Input: dimensioned drawing with shaded views. Units: mm. Origin: part minimum x, y, z. A direction names the side the tool comes from. Round coordinates to 2 decimals unless told otherwise and drop trailing zeros. Order: outer loops, then holes, each group sorted by start corner. A loop starts at its lowest first (then second) coordinate and runs counter-clockwise, first axis right, second up.
Item 1: First-contact query: pin 1 (6 mm diameter, centred on y = 36, z = 19.5, fed in from -X); pin 2 (1.5 mm diameter, centred on x = 41, z = 11.5, fed in from +Y); pin 3 (10 mm diameter, centred on y = 36.5, z = 24.5, fed in from +X); pin 4 (10.5 mm diameter, centred on x = 21.5, z = 13, fed in from +Y). Flat tips, straight axial feed; report the tip coordinate or a pass-through.
Item 2: Cut plane B-B on x = 50. Output: boundary loops of the cut face in (y, z).
Item 3: Mould query, pull axis Z, two halves, no side actions, for the marked faces 1, 2, 3 and 4. Classes: released by +Z, released by -Z, zero draft, split by the parting line, or undercut.
Item 4: Reachability of the marked faces 5, 6 and 7 from +Z, -Z, +X, -X, +Y, -Y: full face, straight path, thin tool, end or side. Return the list, or none.
Item 5: Line query: L1, parallel to Y at x = 50, z = 37; L2, parallel to Z at x = 56.5, y = 11.5; L3, parallel to X at y = 50, z = 35. Output: solid intervals per line, ascending.
Item 6: Cut plane A-A on y = 50. Output: boundary loops of the cut face in (x, z).
Item 7: Cut plane D-D on y = 39.5. Output: boundary loops of the cut face in (x, z).
Item 8: Cut plane C-C on z = 36.5. Output: boundary loops of the cut face in (x, y), then the cut area to 3 significant figures.
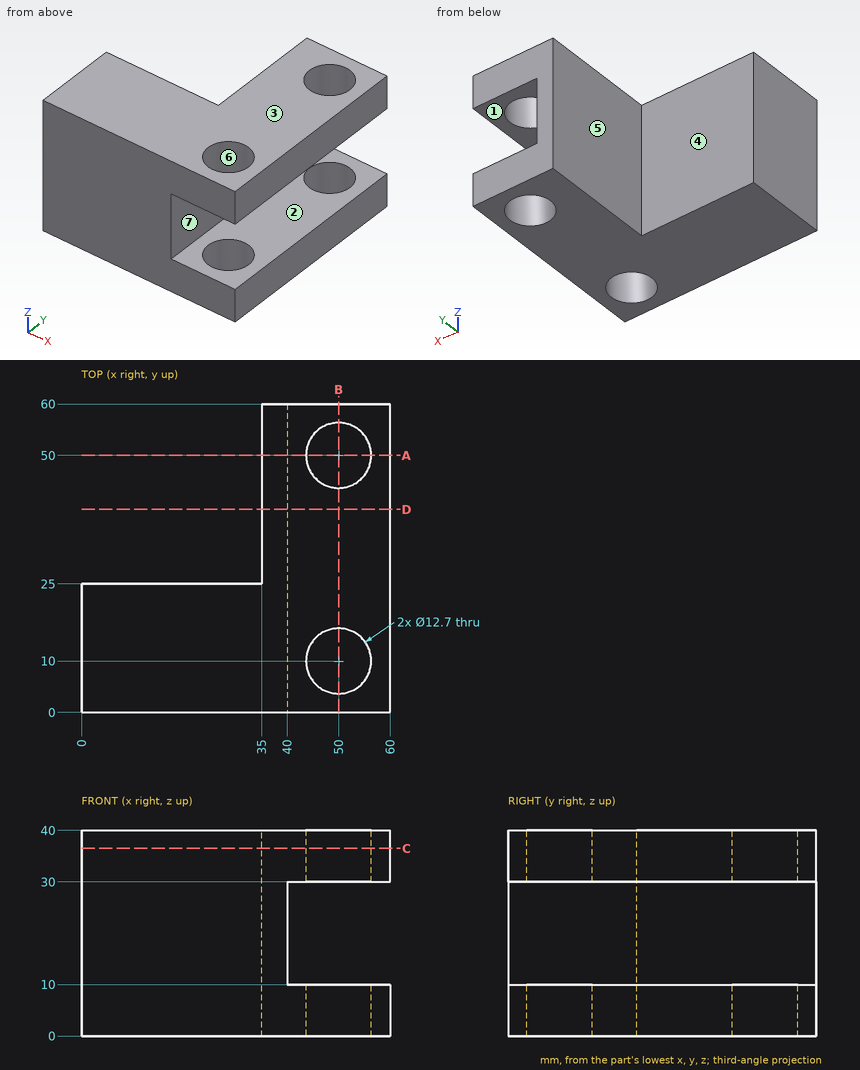
From the geometry:
1. pin 1: stops at x = 35
1. pin 2: passes through
1. pin 3: stops at x = 40
1. pin 4: stops at y = 25
2. outline: (0, 0) - (3.65, 0) - (3.65, 10) - (0, 10) - close; (0, 30) - (3.65, 30) - (3.65, 40) - (0, 40) - close; (16.35, 0) - (43.65, 0) - (43.65, 10) - (16.35, 10) - close; (16.35, 30) - (43.65, 30) - (43.65, 40) - (16.35, 40) - close; (56.35, 0) - (60, 0) - (60, 10) - (56.35, 10) - close; (56.35, 30) - (60, 30) - (60, 40) - (56.35, 40) - close
3. face 1: undercut
3. face 2: undercut
3. face 3: released by +Z
3. face 4: zero draft
4. face 5: +Z, -Z, -X, +Y
4. face 6: +Z, -Z
4. face 7: +X, +Y, -Y
5. L1: y = 0 to 3.65, 16.35 to 43.65, 56.35 to 60
5. L2: z = 0 to 10, 30 to 40
5. L3: x = 35 to 43.65, 56.35 to 60
6. outline: (35, 0) - (43.65, 0) - (43.65, 10) - (40, 10) - (40, 30) - (43.65, 30) - (43.65, 40) - (35, 40) - close; (56.35, 0) - (60, 0) - (60, 10) - (56.35, 10) - close; (56.35, 30) - (60, 30) - (60, 40) - (56.35, 40) - close
7. outline: (35, 0) - (60, 0) - (60, 10) - (40, 10) - (40, 30) - (60, 30) - (60, 40) - (35, 40) - close
8. outline: (0, 0) - (60, 0) - (60, 60) - (35, 60) - (35, 25) - (0, 25) - close; hole circle Ø12.7 at (50, 10); hole circle Ø12.7 at (50, 50)
8. area: 2,120 mm2
